```python
from build123d import *

# Parameters (mm, degrees)
PAD_DEPTH       = 125
PAD001_DEPTH    = 2
PAD002_DEPTH    = 2
SKETCH002_R     = 2.75
POCKET_DEPTH    = 125.001
POCKET001_DEPTH = 125.001
SKETCH004_W     = 12
SKETCH004_H     = 1.0604
POCKET002_DEPTH = 125.001
PAD003_DEPTH    = 2
SKETCH006_R     = 0.5
POCKET003_DEPTH = 125.001


with BuildPart() as part:
    # DWire → Pad (new body)
    with BuildSketch(Plane.XY):
        Polygon((38.0164, 0.396), (40, 0.042), (40, -0.042), (37.9836, -0.1408), (35.9732, -0.2376), (31.9612, -0.4296), (27.9592, -0.6204), (23.966, -0.8096), (19.9804, -0.9872), (16, -1.1348), (12.05, -1.25), (10.0744, -1.292), (8.0956, -1.3104), (6.1112, -1.2908), (4.116, -1.2064), (3.1132, -1.1236), (2.1032, -0.9928), (1.0812, -0.7708), (0.5608, -0.5792), (0, 0), (0.4392, 0.6776), (0.9188, 0.9644), (1.8968, 1.368), (2.8868, 1.6676), (3.884, 1.9064), (5.8888, 2.266), (7.9044, 2.5104), (9.9256, 2.6672), (11.95, 2.75), (16, 2.7348), (20.0196, 2.5424), (24.034, 2.232), (28.0408, 1.8204), (32.0388, 1.3184), (36.0268, 0.7264), align=None)
    extrude(amount=PAD_DEPTH)

    # Sketch → Pad001 (new body)
    with BuildSketch(Plane.XY.offset(125)):
        with BuildLine():
            Line((11.95, 2.75), (-14, 2.75))
            ThreePointArc((-14, 2.75), (-20.357544, 0.729), (-14, -1.292))
            Line((10.0744, -1.292), (-14, -1.292))
            Line((11.95, 2.75), (10.0744, -1.292))
        make_face()
    extrude(amount=-PAD001_DEPTH)

    # Sketch001 → Pad002 (new body)
    with BuildSketch(Plane(origin=(0, 0, 0), x_dir=(1, 0, 0), z_dir=(0, 0, -1))):
        with BuildLine():
            Line((8.0956, 1.3104), (11.95, -2.75))
            Line((11.95, -2.75), (-14, -2.75))
            ThreePointArc((-14, 1.3104), (-20.351015, -0.7198), (-14, -2.75))
            Line((8.0956, 1.3104), (-14, 1.3104))
        make_face()
    extrude(amount=-PAD002_DEPTH)

    # Sketch002 → Pocket (cut, through all)
    with BuildSketch(Plane(origin=(0, 0, 0), x_dir=(1, 0, 0), z_dir=(0, 0, -1))):
        with Locations((-16.851015, -0.7198)):
            Circle(SKETCH002_R)
    extrude(amount=-POCKET_DEPTH, mode=Mode.SUBTRACT)

    # Sketch003 → Pocket001 (cut, through all)
    with BuildSketch(Plane.XY.offset(125)):
        Polygon((28, 0.27625), (26.76025, 0.4975), (25.51675, 0.704), (23.02425, 1.074), (20.5255, 1.38775), (18.02125, 1.645), (15.51225, 1.839), (13, 1.95925), (10.46875, 1.96875), (9.2035, 1.917), (7.94025, 1.819), (6.6805, 1.66625), (5.4275, 1.4415), (4.80425, 1.29225), (4.1855, 1.105), (3.57425, 0.85275), (3.2745, 0.6735), (3, 0.25), (3.3505, -0.112), (3.67575, -0.23175), (4.3145, -0.3705), (4.94575, -0.45225), (5.5725, -0.504), (6.8195, -0.55675), (8.05975, -0.569), (9.2965, -0.5575), (10.53125, -0.53125), (13, -0.45925), (15.48775, -0.367), (17.97875, -0.256), (20.4745, -0.13775), (22.97575, -0.0185), (25.48325, 0.1015), (26.73975, 0.162), (28, 0.22375), align=None)
    extrude(amount=-POCKET001_DEPTH, mode=Mode.SUBTRACT)

    # Sketch004 → Pocket002 (cut, through all)
    with BuildSketch(Plane(origin=(0, 0, 0), x_dir=(1, 0, 0), z_dir=(0, 0, -1))):
        with Locations((-7, -0.7198)):
            Rectangle(SKETCH004_W, SKETCH004_H)
    extrude(amount=-POCKET002_DEPTH, mode=Mode.SUBTRACT)

    # Sketch005 → Pad003 (new body)
    with BuildSketch(Plane(origin=(0, 0, 0), x_dir=(1, 0, 0), z_dir=(0, 0, -1))):
        Polygon((33, 0), (40, 0), (33, 7), align=None)
    extrude(amount=-PAD003_DEPTH)

    # Sketch006 → Pocket003 (cut, through all)
    with BuildSketch(Plane(origin=(0, 0, 0), x_dir=(1, 0, 0), z_dir=(0, 0, -1))):
        with Locations((34, 4.5)):
            Circle(SKETCH006_R)
    extrude(amount=-POCKET003_DEPTH, mode=Mode.SUBTRACT)


solid = part.part
```
Check sheet for the modelled part. Datum: model origin and axes. Units: mm. A direction names the side the tool comes from. Round coordinates to 2 decimals unless told otherwise and drop trailing zeros. Loops run counter-clockwise (first coordinate to the right, second up) from the corner with the lowest first, then second, coordinate; pieces in that order, holes last. Notation, with made-up numbers: (25, -1.5) - (36, -1.5) arc R10 ccw to (36, 17.5) - close; hole circle Ø2 at (71.5, 0). An arc over 180 degrees is marked (long way). Answer as a JSON object with one key per item and string values. Group by question number.
Q1. Mould release check, pull along X, two halves, no side actions. Record for faces 1 (the face through (5, 2, 125)), 2 (the face through (34.005, 1.027, 61.625)), 3 (the face through (16.78, 1.74, 63.38)): released by +X, released by -X, zero draft, split by the parting line, or undercut.
Q2. Set-up check for faces 4 (the face through (37, -3, 1)), 5 (the face through (19.291, 1.515, 63.375)): record each of +Z, -Z, +X, -X, +Y, -Y from which the full face is reachable in a straight line by a thin tool's end or side.
Q3. Sectioned sample at A-A, the plane x = -10. Enter the section's corners in (y, z).
Q4. Scan lines: line 1 along Z through (x, y) = (-14.5, 2.75); line 2 along Y through (x, z) = (20.5, 69); line 3 along Y through (x, z) = (10.5, 71.5). Record each from-to range of solid material in increasing order. Write a range as [from, to].
Q5. Gauge pin test, flat ends, axial feed: P1, Ø1.6, axis at x = -5, z = 123.5, coming from the +Y side; P2, Ø1.6, axis at x = 0, z = 124, coming from the +Y side; P3, Ø12, axis at x = 33, z = 104, coming from the -Y side; P4, Ø1, axis at y = -2.5, z = 112.5, coming from the +X side. Record the tip position at first contact, or that the pin passes through.
Solution:
{
 "1": {"face 1": "zero draft", "face 2": "released by +X", "face 3": "undercut"},
 "2": {"face 4": "+Z, -Z, +X, -Y", "face 5": "+Z, -Z"},
 "3": {"outline": "(-1.31, 0) - (0.19, 0) - (0.19, 2) - (-1.31, 2) - close; (-1.29, 123) - (0.19, 123) - (0.19, 125) - (-1.29, 125) - close; (1.25, 0) - (2.75, 0) - (2.75, 2) - (1.25, 2) - close; (1.25, 123) - (2.75, 123) - (2.75, 125) - (1.25, 125) - close"},
 "4": {"line 1": "z = [0, 2], [123, 125]", "line 2": "y = [-0.96, -0.14], [1.39, 2.51]", "line 3": "y = [-1.28, -0.53], [1.97, 2.69]"},
 "5": {"P1": "stops at y = 2.75", "P2": "stops at y = 2.75", "P3": "stops at y = -0.67", "P4": "passes through"}
}
